Design review of the part built by this model. Coordinates are the model's own, in mm. Face numbers are marked on the shaded views. A direction names the side the tool comes from. Round coordinates to 2 decimals unless told otherwise and drop trailing zeros. Loops run counter-clockwise (first coordinate to the right, second up) from the corner with the lowest first, then second, coordinate; pieces in that order, holes last. Notation, with made-up numbers: M 21,58 L 45,58 A17 ccw 45,86 Z; hole C 75.25,23 d7. An arc over 180 degrees is marked long. One line per item, written item: value. Start each with the question number.
Item 1: Clearance check with flat-ended pins moving along their axes: pin 1 (11.5 mm diameter, centred on x = 23.5, z = 49, fed in from -Y); pin 2 (14.5 mm diameter, centred on x = 57.64, y = -35.87, fed in from +Z). State where each tip first meets the part, or that it passes through.
Item 2: We need section A-A (x = 27). Write out the cut boundary in (y, z), then the cut area to 3 significant figures.
Item 3: We need section B-B (y = 28). Write out the cut boundary in (x, z).
Item 4: For the marked faces 5, 6 and 7, list the 3-axis set-ups (+Z, -Z, +X, -X, +Y, -Y) from which the entire face can be reached by the end or side of a thin tool; tool diameter is ignored.
Item 5: For line 1 along X through (y, z) = (-36, 13.5); line 2 along Y through (x, z) = (73, 60); line 3 along Z through (x, y) = (15, -46), list the stretches that pass through material, from the lowest coordinate up.
Item 6: We need section C-C (x = 55). Write out the cut boundary in (y, z).
Item 7: We need section D-D (z = 46). Write out the cut boundary in (x, y).
Item 8: Mouldability with a two-part tool opening along Z and no side actions: class the marked faces 1, 2, 3 and 4 as released by +Z, released by -Z, zero draft, split by the parting line, or undercut.
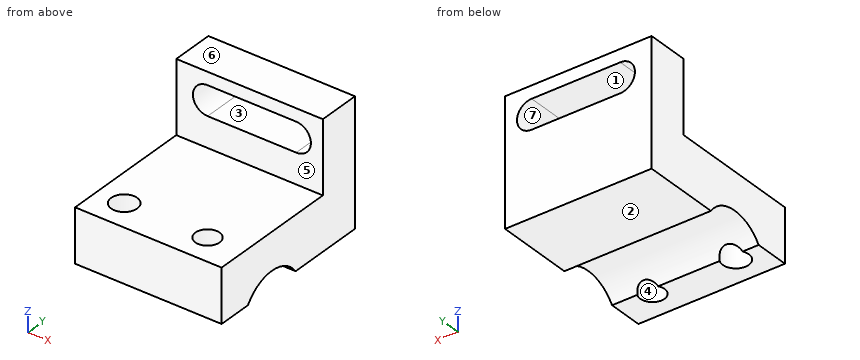
from build123d import *

# Parameters (mm, degrees)
F1_DEPTH = 76.2
F2_R     = 6.778033
F2_R_2   = 6.285837
F3_DEPTH = 63.246
F5_DEPTH = 25.4


with BuildPart() as f1:
    # F0 (on Right) → F1 (new body)
    with BuildSketch(Plane.YZ):
        with BuildLine():
            ThreePointArc((-32.663602, 0), (-16.331801, 8.548074), (0, 0))
            Line((0, 0), (18.621311, 0))
            Line((18.621311, 0), (40.600557, 0))
            Line((40.600557, 0), (40.600557, 65.327212))
            Line((40.600557, 65.327212), (18.621311, 65.327212))
            Line((18.621311, 65.327212), (18.621311, 27.779331))
            Line((18.621311, 27.779331), (-50.674375, 27.779331))
            Line((-50.674375, 27.779331), (-50.674375, 0))
            Line((-50.674375, 0), (-32.663602, 0))
        make_face()
    extrude(amount=F1_DEPTH)

    # F2 (on face) → F3 (cut)
    with BuildSketch(Plane.XY.offset(27.779331)):
        with Locations((14.289155, -35.868905)):
            Circle(F2_R)
        with Locations((57.637118, -35.868905)):
            Circle(F2_R_2)
    extrude(amount=-F3_DEPTH, mode=Mode.SUBTRACT)

    # F4 (on face) → F5 (cut)
    with BuildSketch(Plane(origin=(0, 40.600557, 0), x_dir=(-1, 0, 0), z_dir=(0, 1, 0))):
        with BuildLine():
            Line((-16.286157, 58.71784), (-62.371738, 58.71784))
            ThreePointArc((-62.371738, 58.71784), (-69.991738, 51.09784), (-62.371738, 43.47784))
            Line((-62.371738, 43.47784), (-16.286157, 43.47784))
            ThreePointArc((-16.286157, 43.47784), (-8.666157, 51.09784), (-16.286157, 58.71784))
        make_face()
    extrude(amount=-F5_DEPTH, mode=Mode.SUBTRACT)


solid = f1.part
A:
1. pin 1: y = 18.62
1. pin 2: z = 27.78
2. outline: M -50.67,0 L -32.66,0 A19.88 cw 0,0 L 40.6,0 L 40.6,43.48 L 18.62,43.48 L 18.62,27.78 L -50.67,27.78 Z; M 18.62,58.72 L 40.6,58.72 L 40.6,65.33 L 18.62,65.33 Z
2. area: 2,830 mm2
3. outline: M 0,0 L 76.2,0 L 76.2,65.33 L 0,65.33 Z; hole M 16.29,43.48 L 62.37,43.48 A7.62 ccw 62.37,58.72 L 16.29,58.72 A7.62 ccw Z
4. face 5: +Z, +X, -X, -Y
4. face 6: +Z, +X, -X, +Y, -Y
4. face 7: +Y, -Y
5. line 1: 0 to 7.51, 21.07 to 51.35, 63.92 to 76.2
5. line 2: 18.62 to 40.6
5. line 3: 0 to 27.78
6. outline: M -50.67,0 L -41.57,0 L -41.57,27.78 L -50.67,27.78 Z; M -30.16,2.95 A19.88 cw 0,0 L 40.6,0 L 40.6,43.48 L 18.62,43.48 L 18.62,27.78 L -30.16,27.78 Z; M 18.62,58.72 L 40.6,58.72 L 40.6,65.33 L 18.62,65.33 Z
7. outline: M 0,18.62 L 10.62,18.62 L 10.62,40.6 L 0,40.6 Z; M 68.04,18.62 L 76.2,18.62 L 76.2,40.6 L 68.04,40.6 Z
8. face 1: undercut
8. face 2: released by -Z
8. face 3: undercut
8. face 4: zero draft
